Can you work these out from the model? Positions are in its coordinate system, mm. Give positions to 0.01 mm unless a question says otherwise; leave off trailing zeros. Write each loop counter-clockwise with the first axis right and the second up, starting at its lowest first coordinate (ties: lowest second). Pieces come first, ordered by that corner, then holes.
1. Suppose I cut it at D-D (x = 0.95). Please give me the cut outline in (y, z).
2. Suppose I cut it at A-A (y = 0). Please give me the cut outline in (x, z) (3 decimals).
3. Thinking about a two-plate mould opening in Z: for faces 1 (the cylindrical face through (1.63, 2.98, -0.94)), 2 (the cylindrical face through (0.987, 3.233, 1.341)), which applies, pulls with the +Z half, pulls with the -Z half, needs draft (parallel to the pull), parting line crosses it, or undercut?
4. If I drill on probe 1 along Z at (x, y) = (0.6, 0) (3 decimals); probe 2 along Y at (x, z) = (1.6, 0.75), over which ranges is the centre line in solid material (lowest first)?
5. Suppose I cut it at C-C (x = 1.75). Please give me the cut outline in (y, z) (3 decimals).
```python
from build123d import *


with BuildPart() as part:
    # Sketch1 → Revolve1 (revolve)
    with BuildSketch(Plane.XY):
        with BuildLine():
            Line((0, 3.4), (0, 3.125))
            Line((0, 3.125), (0.751253141, 3.125))
            ThreePointArc((0.751253141, 3.125), (1, 3.2), (1.248746859, 3.125))
            Line((1.248746859, 3.125), (2, 3.125))
            Line((2, 3.125), (2, 3.4))
            ThreePointArc((2, 3.4), (1.970710678, 3.470710678), (1.9, 3.5))
            Line((1.9, 3.5), (0.1, 3.5))
            ThreePointArc((0.1, 3.5), (0.029289322, 3.470710678), (0, 3.4))
        make_face()
    revolve(axis=Axis((2, 0, 0), (-1, 0, 0)))


solid = part.part
```
Checks:
1. outline: circle Ø7 at (0, 0); hole circle Ø6.39 at (0, 0)
2. outline: (0, -3.4) arc R0.1 ccw to (0.1, -3.5) - (1.9, -3.5) arc R0.1 ccw to (2, -3.4) - (2, -3.125) - (1.249, -3.125) arc R0.45 cw to (0.751, -3.125) - (0, -3.125) - close; (0, 3.125) - (0.751, 3.125) arc R0.45 cw to (1.249, 3.125) - (2, 3.125) - (2, 3.4) arc R0.1 ccw to (1.9, 3.5) - (0.1, 3.5) arc R0.1 ccw to (0, 3.4) - close
3. face 1: undercut
3. face 2: parting line crosses it
4. probe 1: z = -3.5 to -3.125, 3.125 to 3.5
4. probe 2: y = -3.42 to -3.03, 3.03 to 3.42
5. outline: circle Ø7 at (0, 0); hole circle Ø6.25 at (0, 0)
